Part model, mm, in its own coordinate system. Face numbers are marked on the shaded views. Coordinates: 2 decimals unless noted, no trailing zeros. Order: outer loops, then holes, each group sorted by start corner. A loop starts at its lowest first (then second) coordinate and runs counter-clockwise, first axis right, second up. Notation, with made-up numbers: (39.25, 50.5) - (74.25, 50.5) arc R24 cw to (74.25, 66.5) - close; hole circle Ø10 at (6.5, 80.5). An arc over 180 degrees is marked (long way). Use a Markdown table: item, result. Add a question column.
1) Saw through at B-B on x = 81. List the corners of the cut face in (y, z).
2) Saw through at A-A on y = -80.5. Count the separate pieces of the cut face and the enclosed holes in it, then the cut area to 3 significant figures.
3) Saw through at D-D on x = 418.5. List the corners of the cut face in (y, z), then the cut area to 3 significant figures.
4) Drop flat-ended pins along their axis: P1, Ø10, axis at y = -58.5, z = -33.5, coming from the +X side; P2, Ø6.5, axis at x = 315.5, y = 7.5, coming from the -Z side; P3, Ø6.5, axis at y = -82, z = -242.5, coming from the +X side; P4, Ø12, axis at x = 198, y = -14.5, coming from the -Z side. Give the stop position or say it passes through.
5) Two-plate mould, pull along X, no slides. Class the marked faces 1 and 2: +X half, -X half, draft (parallel to the pull), parting line (faces both ways), or undercut.
6) Wall check: L1, parallel to Z at x = 215.9, y = 0.4 (1 decimal); L2, parallel to X at y = -23, z = -22; L3, parallel to X at y = 24.25, z = -12.7 (1 decimal). Give the ranges that are in metal, low to high. Write a range as [from, to].
7) Saw through at C-C on z = -35. List the corners of the cut face in (x, y).
Autodesk Inventor part; units mm, degrees
ref_plane "YZ Plane" through (0, 0, 0) normal (1, 0, 0) x (0, 1, 0)
ref_plane "XZ Plane" through (0, 0, 0) normal (0, 1, 0) x (-1, 0, 0)
ref_plane "XY Plane" through (0, 0, 0) normal (0, 0, 1) x (1, 0, 0)
sketch "Sketch1" plane through (0, 0, 0) normal (1, 0, 0) x (0, 1, 0)
  line L0 (0, 0) -> (25.4, 0)
  line L1 (25.4, 0) -> (25.4, -25.4)
  line L2 (25.4, -25.4) -> (0, -25.4)
  line L3 (0, -25.4) -> (0, 0)
  line L4 (1.5875, -1.5875) -> (23.8125, -1.5875)
  line L5 (23.8125, -1.5875) -> (23.8125, -23.8125)
  line L6 (23.8125, -23.8125) -> (1.5875, -23.8125)
  line L7 (1.5875, -23.8125) -> (1.5875, -1.5875)
  dimension "d0" = 25.4
  dimension "d1" = 1.5875
  dimension "d2" = 1.5875
  dimension "d3" = 1.5875
  dimension "d4" = 1.5875
extrude "Extrusion1" add sketch "Sketch1" along normal blind 431.8
sketch "Sketch2" plane through (0, 0, -25.4) normal (0, 0, -1) x (-1, 0, 0)
  line L0 (0, 25.4) -> (0, 0)
  line L1 (0, 25.4) -> (-431.8, 25.4)
  line L2 (0, 0) -> (-431.8, 0) construction
  line L3 (-228.6, 0) -> (-203.2, 0)
  line L4 (-203.2, 0) -> (-203.2, 25.4)
  line L5 (-203.2, 25.4) -> (-228.6, 25.4)
  line L6 (-228.6, 25.4) -> (-228.6, 0)
  line L7 (-215.9, 25.4) -> (-215.9, 0) construction
  line L8 (-227.0125, 1.5875) -> (-204.7875, 1.5875)
  line L9 (-204.7875, 1.5875) -> (-204.7875, 23.8125)
  line L10 (-204.7875, 23.8125) -> (-227.0125, 23.8125)
  line L11 (-227.0125, 23.8125) -> (-227.0125, 1.5875)
  line L12 (-227.0125, 1.5875) -> (-204.7875, 23.8125) construction
  line L13 (-204.7875, 1.5875) -> (-227.0125, 23.8125) construction
  point P0 (-215.9, 12.7)
  dimension "d7" = 25.4
  dimension "d9" = 12.7
  dimension "d10" = 215.9
  dimension "d11" = 1.5875
  dimension "d12" = 1.5875
  dimension "d13" = 1.5875
  dimension "d14" = 1.5875
extrude "Extrusion2" add sketch "Sketch2" along normal blind 203.2
sketch "Sketch3" plane through (203.2, 0, -25.4) normal (-1, 0, 0) x (0, 0, 1)
  line L0 (0, 25.4) -> (0, 0)
  line L1 (0, 25.4) -> (-203.2, 25.4)
  line L2 (0, 0) -> (-203.2, 0)
  line L3 (-127, 0) -> (-101.6, 0)
  line L4 (-101.6, 0) -> (-101.6, 25.4)
  line L5 (-101.6, 25.4) -> (-127, 25.4)
  line L6 (-127, 25.4) -> (-127, 0)
  line L7 (-114.3, 25.4) -> (-114.3, 0) construction
  line L8 (-125.4125, 1.5875) -> (-103.1875, 1.5875)
  line L9 (-103.1875, 1.5875) -> (-103.1875, 23.8125)
  line L10 (-103.1875, 23.8125) -> (-125.4125, 23.8125)
  line L11 (-125.4125, 23.8125) -> (-125.4125, 1.5875)
  point P0 (25.4, 0)
  dimension "d17" = 25.4
  dimension "d19" = 12.7
  dimension "d20" = 114.3
  dimension "d21" = 1.5875
  dimension "d22" = 1.5875
  dimension "d23" = 1.5875
  dimension "d24" = 1.5875
extrude "Extrusion3" add sketch "Sketch3" along normal blind 203.2 contours L4 L2 L6 L1
sketch "Sketch4" plane through (0, 25.4, 0) normal (0, 1, 0) x (1, 0, 0)
  line L0 (0, 0) -> (0, 25.4)
  line L1 (431.8, 25.4) -> (431.8, 0)
  line L2 (203.2, 228.6) -> (228.6, 228.6)
  line L3 (0, 127) -> (-25.4, 127)
  line L4 (-25.4, 127) -> (-25.4, 152.4)
  line L5 (-25.4, 152.4) -> (0, 152.4)
  line L6 (0, 152.4) -> (0, 127)
  line L7 (0, 0) -> (-25.4, 0)
  line L8 (-25.4, 0) -> (-25.4, 25.4)
  line L9 (-25.4, 25.4) -> (0, 25.4)
  line L10 (0, 25.4) -> (0, 0)
  line L11 (431.8, 0) -> (457.2, 0)
  line L12 (457.2, 0) -> (457.2, 25.4)
  line L13 (457.2, 25.4) -> (431.8, 25.4)
  line L14 (431.8, 25.4) -> (431.8, 0)
  line L15 (203.2, 228.6) -> (206.375, 228.6)
  line L16 (-23.8125, 128.5875) -> (-1.5875, 128.5875)
  line L17 (-1.5875, 128.5875) -> (-1.5875, 150.8125)
  line L18 (-1.5875, 150.8125) -> (-23.8125, 150.8125)
  line L19 (-23.8125, 150.8125) -> (-23.8125, 128.5875)
  line L20 (-23.8125, 1.5875) -> (-1.5875, 1.5875)
  line L21 (-1.5875, 1.5875) -> (-1.5875, 23.8125)
  line L22 (-1.5875, 23.8125) -> (-23.8125, 23.8125)
  line L23 (-23.8125, 23.8125) -> (-23.8125, 1.5875)
  line L24 (204.7875, 234.8076) -> (204.7875, 234.8076)
  line L25 (433.3875, 1.5875) -> (455.6125, 1.5875)
  line L26 (455.6125, 1.5875) -> (455.6125, 23.8125)
  line L27 (455.6125, 23.8125) -> (433.3875, 23.8125)
  line L28 (433.3875, 23.8125) -> (433.3875, 1.5875)
  line L29 (203.2, 228.6) -> (228.6, 228.6)
  line L30 (228.6, 228.6) -> (228.6, 254)
  line L31 (228.6, 254) -> (203.2, 254)
  line L32 (203.2, 254) -> (203.2, 228.6)
  line L33 (204.7875, 230.1875) -> (227.0125, 230.1875)
  line L34 (227.0125, 230.1875) -> (227.0125, 252.4125)
  line L35 (227.0125, 252.4125) -> (204.7875, 252.4125)
  line L36 (204.7875, 252.4125) -> (204.7875, 230.1875)
  dimension "d27" = 25.4
  dimension "d28" = 25.4
  dimension "d29" = 25.4
  dimension "d33" = 25.4
  dimension "d34" = 25.4
  dimension "d35" = 1.5875
  dimension "d36" = 1.5875
  dimension "d37" = 1.5875
  dimension "d39" = 1.5875
  dimension "d40" = 1.5875
  dimension "d41" = 1.5875
  dimension "d42" = 1.5875
  dimension "d43" = 1.5875
  dimension "d44" = 1.5875
  dimension "d45" = 1.5875
  dimension "d46" = 1.5875
  dimension "d47" = 1.5875
  dimension "d48" = 1.5875
  dimension "d49" = 1.5875
  dimension "d50" = 1.5875
  dimension "d51" = 1.5875
extrude "Extrusion4" add sketch "Sketch4" against normal blind 152.4
sketch "Sketch5" plane through (203.2, 25.4, -25.4) normal (0, 1, 0) x (1, 0, 0)
  line L0 (-228.6, -25.4) -> (254, -25.4)
  line L1 (228.6, -23.8125) -> (228.6, -1.5875)
  point P0 (-203.2, -25.4)
  point P1 (12.7, -12.7)
  dimension "d54" = 12.7
  dimension "d55" = 215.9
hole "Hole1" at (215.9, 25.4, -12.7) direction (0, -1, 0) diameter 6.35 depth 25.4 tip angle 118
properties part number "TopSupportV3"
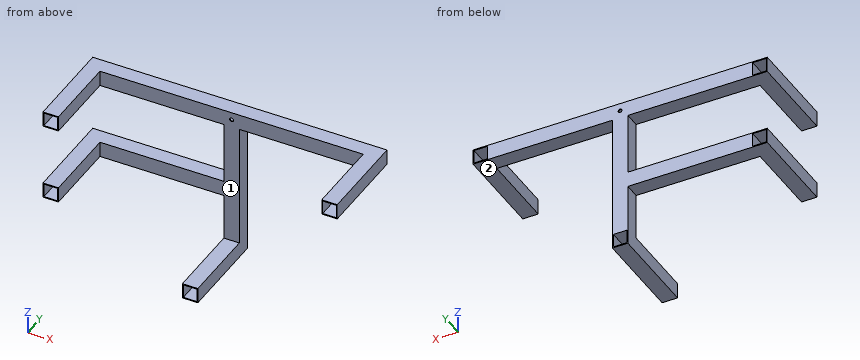
Results are:
| question | item | result |
|---|---|---|
| 1 | outline | (0, -152.4) - (25.4, -152.4) - (25.4, -127) - (0, -127) - close; (0, -25.4) - (25.4, -25.4) - (25.4, 0) - (0, 0) - close; hole (1.59, -150.81) - (23.81, -150.81) - (23.81, -128.59) - (1.59, -128.59) - close; hole (1.59, -23.81) - (23.81, -23.81) - (23.81, -1.59) - (1.59, -1.59) - close |
| 2 | separate pieces | 4 |
| 2 | enclosed holes | 4 |
| 2 | area | 605 mm2 |
| 3 | outline | (0, -25.4) - (25.4, -25.4) - (25.4, 0) - (0, 0) - close; hole (1.59, -23.81) - (23.81, -23.81) - (23.81, -1.59) - (1.59, -1.59) - close |
| 3 | area | 151 mm2 |
| 4 | P1 | through |
| 4 | P2 | z = -25.4 |
| 4 | P3 | x = 228.6 |
| 4 | P4 | z = -254 |
| 5 | face 1 | undercut |
| 5 | face 2 | draft |
| 6 | L1 | [-254, -252.4], [-230.2, -15.9], [-9.5, 0] |
| 6 | L2 | [-25.4, -23.81], [-1.59, 0], [431.8, 433.39], [455.61, 457.2] |
| 6 | L3 | [-25.4, -23.8], [-1.6, 212.7], [219.1, 433.4], [455.6, 457.2] |
| 7 | outline | (203.2, 0) - (228.6, 0) - (228.6, 25.4) - (203.2, 25.4) - close; hole (204.79, 1.59) - (227.01, 1.59) - (227.01, 23.81) - (204.79, 23.81) - close |
